from build123d import *

# Parameters (mm, degrees)
BOSS_EXTRUDE1_DEPTH = 5
SKETCH1_3_W         = 10
SKETCH1_3_H         = 5
BOSS_EXTRUDE2_DEPTH = 9
SKETCH2_W           = 40
SKETCH2_H           = 3.955098896
BOSS_EXTRUDE4_DEPTH = 28
FILLET1_R           = 2
SKETCH6_R           = 1.6
CUT_EXTRUDE1_DEPTH  = 3.955098897
FILLET2_R           = 1


with BuildPart() as part:
    # Sketch1 → Boss-Extrude1 (new body)
    with BuildSketch(Plane(origin=(0, 0, 0), x_dir=(1, 0, 0), z_dir=(0, 1, 0))):
        Polygon((-4.61462686, -18.720861087), (-14.61462686, -18.720861087), (-14.61462686, -25.920861087), (-34.61462686, -25.920861087), (-34.61462686, -18.720861087), (-44.61462686, -18.720861087), (-44.61462686, -35.875959983), (-4.61462686, -35.875959983), align=None)
    extrude(amount=BOSS_EXTRUDE1_DEPTH)

    # Sketch1<3> → Boss-Extrude2 (add)
    with BuildSketch(Plane(origin=(0, 0, 0), x_dir=(1, 0, 0), z_dir=(0, 1, 0))):
        with Locations((-39.61462686, -21.220861087)):
            Rectangle(SKETCH1_3_W, SKETCH1_3_H)
        with Locations((-9.61462686, -21.220861087)):
            Rectangle(SKETCH1_3_W, SKETCH1_3_H)
    extrude(amount=BOSS_EXTRUDE2_DEPTH)

    # Sketch2 → Boss-Extrude4 (add)
    with BuildSketch(Plane(origin=(0, 5, 0), x_dir=(1, 0, 0), z_dir=(0, 1, 0))):
        with Locations((-24.61462686, -33.898410535)):
            Rectangle(SKETCH2_W, SKETCH2_H)
    extrude(amount=BOSS_EXTRUDE4_DEPTH)

    # Fillet1
    fillet1_edges = [part.edges().sort_by_distance(p)[0] for p in [
        (-34.61462686, 0, 22.320861087),
        (-24.61462686, 0, 25.920861087),
        (-14.61462686, 0, 22.320861087),
        (-9.61462686, 0, 18.720861087),
        (-4.61462686, 0, 27.298410535),
        (-24.61462686, 0, 35.875959983),
        (-44.61462686, 0, 27.298410535),
        (-44.61462686, 4.5, 18.720861087),
        (-34.61462686, 4.5, 18.720861087),
        (-14.61462686, 4.5, 18.720861087),
        (-4.61462686, 4.5, 18.720861087),
        (-4.61462686, 16.5, 35.875959983),
        (-44.61462686, 16.5, 35.875959983),
        (-24.61462686, 5, 25.920861087),
        (-39.61462686, 9, 18.720861087),
        (-44.61462686, 9, 21.220861087),
        (-34.61462686, 9, 21.220861087),
        (-14.61462686, 9, 21.220861087),
        (-4.61462686, 9, 21.220861087),
        (-9.61462686, 9, 18.720861087),
        (-39.61462686, 0, 18.720861087),
    ]]
    fillet(fillet1_edges, radius=FILLET1_R)

    # Sketch6 → Cut-Extrude1 (cut)
    with BuildSketch(Plane(origin=(0, 0, 31.920861087), x_dir=(-1, 0, 0), z_dir=(0, 0, -1))):
        with Locations((24.61462686, 12)):
            Circle(SKETCH6_R)
    extrude(amount=-CUT_EXTRUDE1_DEPTH, mode=Mode.SUBTRACT)

    # Fillet2
    fillet2_edges = [part.edges().sort_by_distance(p)[0] for p in [
        (-23.01462686, 12, 31.920861087),
        (-23.01462686, 12, 35.875959984),
    ]]
    fillet(fillet2_edges, radius=FILLET2_R)


solid = part.part
The model under review builds one solid part; all positions refer to its coordinate system, in mm. A direction names the side the tool comes from. Round coordinates to 2 decimals unless told otherwise and drop trailing zeros. Write each loop counter-clockwise with the first axis right and the second up, starting at its lowest first coordinate (ties: lowest second). Pieces come first, ordered by that corner, then holes. Notation, with made-up numbers: (0.25, 49.25) - (40.25, 49.25) arc R22 ccw to (40.25, 64.25) - close; hole circle Ø7 at (18.5, 54). An arc over 180 degrees is marked (long way). One line per item, written item: value. Start each with the question number.
1. The part is to be moulded in two halves that separate along X. For faces 1 (the face through (-9.66, 0.6, 19.29)), 2 (the face through (-34.615, 4, 23)), 3 (the face through (-44.044, 8.399, 22.2)), 4 (the face through (-5.22, 17.72, 35.31)), say which applies: released by +X, released by -X, zero draft, split by the parting line, or undercut.
2. Consider section A-A on y = 12. Write out the cut boundary in (x, z), and give its area (3 significant figures).
3. Machinability: for faces 5 (the face through (-14.01, 4.46, 19.29)), 6 (the face through (-40, 9, 22)), 7 (the face through (-14.044, 8.399, 22.2)), 8 (the face through (-24.78, 0.6, 26.49)), 9 (the face through (-10, 7, 23.721)), which of the approach directions +Z, -Z, +X, -X, +Y, -Y give a long, thin tool a straight path to every point of the face, cutting with its end or side? Answer none if there is none.
4. Clearance check with flat-ended pins moving along their axes: P1, Ø3.5, axis at x = -10.5, z = 22, coming from the +Y side; P2, Ø4, axis at x = -17.5, z = 25, coming from the -Y side; P3, Ø4, axis at x = -30, z = 27, coming from the +Y side. State where each tip first meets the part, or that it passes through.
5. To check wall thickness, follow L1, parallel to Z at x = -19, y = 14.5; L2, parallel to Y at x = -18, z = 34; L3, parallel to Y at x = -6.5, z = 24.5. State the ranges of each line that lie inside material, in increasing order. Write a range as from..to.
6. Consider section B-B on z = 25. Write out the cut boundary in (x, y).
7. Consider section C-C on x = -34. Write out the cut boundary in (y, z), and give its area (3 significant figures).
8. Consider section D-D on y = 8.5. Write out the cut boundary in (x, z).
Checks:
1. face 1: zero draft
1. face 2: undercut
1. face 3: released by -X
1. face 4: released by +X
2. outline: (-44.61, 31.92) - (-27.21, 31.92) arc R1 ccw to (-26.21, 32.92) - (-26.21, 34.88) arc R1 ccw to (-27.21, 35.88) - (-42.61, 35.88) arc R2 ccw to (-44.61, 33.88) - close; (-23.01, 32.92) arc R1 ccw to (-22.01, 31.92) - (-4.61, 31.92) - (-4.61, 33.88) arc R2 ccw to (-6.61, 35.88) - (-22.01, 35.88) arc R1 ccw to (-23.01, 34.88) - close
2. area: 143 mm^2
3. face 5: -Z, +Y, -Y
3. face 6: -Z, +X, -X, +Y
3. face 7: -Z, +Y
3. face 8: -Z, -Y
3. face 9: +X, -X, +Y
4. P1: stops at y = 9
4. P2: stops at y = 0.22
4. P3: stops at y = 5
5. L1: z = 31.92..35.88
5. L2: y = 0..33
5. L3: y = 0..5
6. outline: (-44.61, 2) arc R2 ccw to (-42.61, 0) - (-36.61, 0) arc R2 ccw to (-34.61, 2) - (-34.61, 5) - (-44.61, 5) - close; (-14.61, 2) arc R2 ccw to (-12.61, 0) - (-6.61, 0) arc R2 ccw to (-4.61, 2) - (-4.61, 5) - (-14.61, 5) - close
7. outline: (0, 27.92) arc R2 ccw to (2, 25.92) - (3, 25.92) arc R2 ccw to (5, 27.92) - (5, 31.92) - (33, 31.92) - (33, 35.88) - (2, 35.88) arc R2 ccw to (0, 33.88) - close
7. area: 158 mm^2
8. outline: (-44.61, 31.92) - (-4.61, 31.92) - (-4.61, 33.88) arc R2 ccw to (-6.61, 35.88) - (-42.61, 35.88) arc R2 ccw to (-44.61, 33.88) - close; (-43.94, 20.72) arc R1.32 ccw to (-42.61, 19.4) - (-36.61, 19.4) arc R1.32 ccw to (-35.29, 20.72) - (-35.29, 23.72) - (-43.94, 23.72) - close; (-13.94, 20.72) arc R1.32 ccw to (-12.61, 19.4) - (-6.61, 19.4) arc R1.32 ccw to (-5.29, 20.72) - (-5.29, 23.72) - (-13.94, 23.72) - close
